```python
from build123d import *

# Parameters (mm, degrees)
SKETCH1_W               = 10
SKETCH1_H               = 647.7
SKETCH2_R               = 3.2
CUT_EXTRUDE1_DEPTH      = 11
CUT_EXTRUDE1_DEPTH_BACK = 11


with BuildPart() as part:
    # Sketch1 → Revolve2 (revolve)
    with BuildSketch(Plane(origin=(0, 0, 0), x_dir=(0, 0, -1), z_dir=(1, 0, 0))):
        with Locations((-5, 323.85)):
            Rectangle(SKETCH1_W, SKETCH1_H)
    revolve(axis=Axis((0, 0, 0), (0, 1, 0)))

    # Sketch2 → Cut-Extrude1 (cut, two sides)
    with BuildSketch(Plane(origin=(0, 0, 0), x_dir=(0, 0, -1), z_dir=(1, 0, 0))) as cut_extrude1_sk:
        with Locations((0, 638.7)):
            Circle(SKETCH2_R)
        with Locations((0, 12)):
            Circle(SKETCH2_R)
    extrude(amount=CUT_EXTRUDE1_DEPTH, mode=Mode.SUBTRACT)
    extrude(cut_extrude1_sk.sketch, amount=-CUT_EXTRUDE1_DEPTH_BACK, mode=Mode.SUBTRACT)


solid = part.part
```
For this review, take the finished solid that the model builds, in its own axes (mm). Coordinates: 2 decimals unless noted, no trailing zeros. Write each loop counter-clockwise with the first axis right and the second up, starting at its lowest first coordinate (ties: lowest second). Pieces come first, ordered by that corner, then holes.
(1) For pin 1 Ø1 at (y, z) = (563, 7) entering from +X; pin 2 Ø6 at (x, y) = (5.5, 431.5) entering from -Z; pin 3 Ø6 at (x, y) = (5.5, 192) entering from +Z, all flat-tipped, find the tip position at first contact; note any pin that passes through.
(2) Add section B-B on y = 197.5. Give the boundary of the cut face in (x, z), then the cut area to 3 significant figures.
(3) Wall thickness on probe 1 along Y at (x, z) = (-4, 0); probe 2 along Y at (x, z) = (-1.75, -1.5); probe 3 along X at (y, z) = (452.5, 1.5): over which ranges is each line inside the solid? List them lowest first.
(4) Add section A-A on z = 0. Give the boundary of the cut face in (x, y), then the cut area to 3 significant figures.
Answer sheet:
1. pin 1: stops at x = 7.6
1. pin 2: stops at z = -9.68
1. pin 3: stops at z = 9.68
2. outline: circle Ø20 at (0, 0)
2. area: 314 mm2
3. probe 1: y = 0 to 8.8, 15.2 to 635.5, 641.9 to 647.7
3. probe 2: y = 0 to 9.17, 14.83 to 635.87, 641.53 to 647.7
3. probe 3: x = -9.89 to 9.89
4. outline: (-10, 0) - (10, 0) - (10, 8.8) - (-10, 8.8) - close; (-10, 15.2) - (10, 15.2) - (10, 635.5) - (-10, 635.5) - close; (-10, 641.9) - (10, 641.9) - (10, 647.7) - (-10, 647.7) - close
4. area: 12,700 mm2
